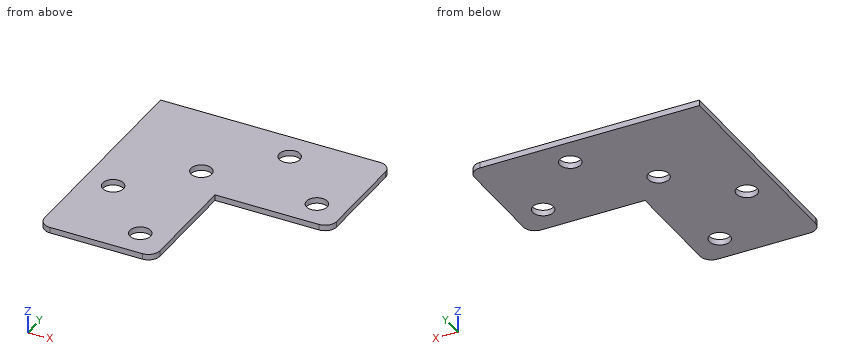
```python
from build123d import *

# Parameters (mm, degrees)
F1_DEPTH = 5
F2_R     = 9
F3_DEPTH = 25
F4_R     = 10


with BuildPart() as f1:
    # F0 (on Top) → F1 (new body)
    with BuildSketch(Plane.XY):
        Polygon((200, 0), (0, 0), (0, -200), (100, -200), (100, -100), (200, -100), align=None)
    extrude(amount=F1_DEPTH)

    # F2 (on face) → F3 (cut)
    with BuildSketch(Plane.XY.offset(5)):
        with Locations((175.000086, -74.999993)):
            Circle(F2_R)
        with Locations((125.000086, -24.999993)):
            Circle(F2_R)
        with Locations((75.000086, -74.999993)):
            Circle(F2_R)
        with Locations((75.000086, -174.999993)):
            Circle(F2_R)
        with Locations((25.000086, -124.999993)):
            Circle(F2_R)
    extrude(amount=-F3_DEPTH, mode=Mode.SUBTRACT)

    # F4
    f4_edges = [f1.edges().sort_by_distance(p)[0] for p in [
        (0, -200, 2.5),
        (100, -200, 2.5),
        (200, -100, 2.5),
        (200, 0, 2.5),
    ]]
    fillet(f4_edges, radius=F4_R)


solid = f1.part
```
Work out the finished part from the listing and answer in its coordinate system (mm). Coordinates: 2 decimals unless noted, no trailing zeros. Loops run counter-clockwise (first coordinate to the right, second up) from the corner with the lowest first, then second, coordinate; pieces in that order, holes last. Notation, with made-up numbers: M 82,-14.75 L 113,-14.75 A8 cw 113,-10.75 Z; hole C 6,60.5 d1. An arc over 180 degrees is marked long. Use CSV: the item, a comma, the result in double quotes. Start each with the question number.
(1) Find section D-D, the plane y = -107.5. Give the vertices of the cut face in (x, z).
(2) Consider line 1 (X direction, y = -67, z = 2.95); line 2 (Y direction, x = 25.5, z = 2.25); line 3 (X direction, y = -78.5, z = 4.2). Determine where each line is inside the solid, lowest interval first.
(3) Given pin 1 Ø16 at (x, y) = (25, -125) entering from +Z; pin 2 Ø2.5 at (y, z) = (-156.5, 1.5) entering from +X; pin 3 Ø1.5 at (x, z) = (158.5, 3) entering from -Y, each flat-ended and moving along its own axis, determine where each tip first touches the part or whether it passes through.
(4) Find section C-C, the plane x = 153.5. Give the vertices of the cut face in (y, z), then the cut area to 3 significant figures.
(5) Find section B-B, the plane x = 20. Give the vertices of the cut face in (y, z).
(6) Find section A-A, the plane z = 2.7. Give the vertices of the cut face in (x, y), then the cut area to 3 significant figures.
Recorded:
1,outline,"M 0,0 L 100,0 L 100,5 L 0,5 Z"
2,line 1,"x = 0 to 70.88, 79.12 to 170.88, 179.12 to 200"
2,line 2,"y = -200 to -133.99, -116.01 to 0"
2,line 3,"x = 0 to 66.71, 83.29 to 166.71, 183.29 to 200"
3,pin 1,"passes through"
3,pin 2,"stops at x = 100"
3,pin 3,"stops at y = -100"
4,outline,"M -100,0 L 0,0 L 0,5 L -100,5 Z"
4,area,"500 mm^2"
5,outline,"M -200,0 L -132.48,0 L -132.48,5 L -200,5 Z; M -117.52,0 L 0,0 L 0,5 L -117.52,5 Z"
6,outline,"M 0,-190 A10 ccw 10,-200 L 90,-200 A10 ccw 100,-190 L 100,-100 L 190,-100 A10 ccw 200,-90 L 200,-10 A10 ccw 190,0 L 0,0 Z; hole C 25,-125 d18; hole C 75,-175 d18; hole C 75,-75 d18; hole C 125,-25 d18; hole C 175,-75 d18"
6,area,"28,600 mm^2"
